Read the model definition and answer for the solid it produces. Units are mm, in the model's axes. Give positions to 0.01 mm unless a question says otherwise; leave off trailing zeros. Order: outer loops, then holes, each group sorted by start corner. A loop starts at its lowest first (then second) coordinate and runs counter-clockwise, first axis right, second up. Notation, with made-up numbers: (-22.75, 74) - (-8.75, 74) arc R18 cw to (-8.75, 89) - close; hole circle Ø4 at (76.5, 62). An arc over 180 degrees is marked (long way). Write each question's results on one line, items separated by ' | '. Start each with the question number.
Q1. Find section C-C on x = 25.5. Give the vertices of the cut face in (y, z).
Q2. Find the intervals of material crossed by line 1 along Z through (x, y) = (-41.5, 1.1); line 2 along X through (y, z) = (0.3, -42); line 3 along X through (y, z) = (1.55, -26), in increasing order. Write a range as from..to.
Q3. Flat-ended cylindrical pins translate along their axes: P1, Ø1, axis at y = 4, z = -29, coming from the -X side; P2, Ø1.5, axis at y = 2, z = -28.5, coming from the +X side; P3, Ø3, axis at x = -17, y = 3.5, coming from the +Z side. Find the tip coordinate at first contact, or state that the pin passes through.
Q4. Find section B-B on z = 38.5. Give the vertices of the cut face in (x, y), and give its area (3 significant figures).
Q5. Find section A-A on y = 3.7. Count the separate pieces of the cut face and the enclosed holes in it, and give its area (3 significant figures).
from build123d import *

# Parameters (mm, degrees)
BOSS_EXTRUDE2_DEPTH = 5
FILLET2_R           = 5
SKETCH4_R           = 2.25
CUT_EXTRUDE1_DEPTH  = 68.360967927


with BuildPart() as part:
    # Sketch3 → Boss-Extrude2 (new body)
    with BuildSketch(Plane(origin=(0, 0, 0), x_dir=(1, 0, 0), z_dir=(0, 1, 0))):
        with BuildLine():
            Line((-32.880465325, -20.152543264), (-39.343121117, -26.615199056))
            ThreePointArc((-39.343121117, -26.615199056), (-37.337514667, -29.36256117), (-35.140434727, -31.95934679))
            ThreePointArc((-35.140434727, -31.95934679), (-32.701976515, -31.519186154), (-31.337572106, -33.587572106))
            ThreePointArc((-31.337572106, -33.587572106), (-31.498791725, -34.423931191), (-31.95934679, -35.140434727))
            ThreePointArc((-31.95934679, -35.140434727), (-29.36256117, -37.337514667), (-26.615199056, -39.343121117))
            Line((-26.615199056, -39.343121117), (-20.152543264, -32.880465325))
            Line((-20.152543264, -32.880465325), (-32.880465325, -20.152543264))
        make_face()
        with BuildLine():
            ThreePointArc((-35.140434727, -31.95934679), (-37.337514667, -29.36256117), (-39.343121117, -26.615199056))
            Line((-39.343121117, -26.615199056), (-42.072853481, -29.344931419))
            ThreePointArc((-42.072853481, -29.344931419), (-43.537319575, -32.880465325), (-42.072853481, -36.415999231))
            Line((-42.072853481, -36.415999231), (-36.415999231, -42.072853481))
            ThreePointArc((-36.415999231, -42.072853481), (-32.880465325, -43.537319575), (-29.344931419, -42.072853481))
            Line((-29.344931419, -42.072853481), (-26.615199056, -39.343121117))
            ThreePointArc((-26.615199056, -39.343121117), (-29.36256117, -37.337514667), (-31.95934679, -35.140434727))
            ThreePointArc((-31.95934679, -35.140434727), (-35.178562364, -35.178562364), (-35.140434727, -31.95934679))
        make_face()
        with BuildLine():
            Line((42.072853481, -29.344931419), (39.343121117, -26.615199056))
            ThreePointArc((39.343121117, -26.615199056), (37.337514667, -29.36256117), (35.140434727, -31.95934679))
            ThreePointArc((35.140434727, -31.95934679), (35.655958059, -32.701976515), (35.837572106, -33.587572106))
            ThreePointArc((35.837572106, -33.587572106), (34.423931191, -35.676352488), (31.95934679, -35.140434727))
            ThreePointArc((31.95934679, -35.140434727), (29.36256117, -37.337514667), (26.615199056, -39.343121117))
            Line((26.615199056, -39.343121117), (29.344931419, -42.072853481))
            ThreePointArc((29.344931419, -42.072853481), (32.880465325, -43.537319575), (36.415999231, -42.072853481))
            Line((36.415999231, -42.072853481), (42.072853481, -36.415999231))
            ThreePointArc((42.072853481, -36.415999231), (43.537319575, -32.880465325), (42.072853481, -29.344931419))
        make_face()
        with BuildLine():
            Line((-20.152543264, 32.880465325), (-26.615199056, 39.343121117))
            ThreePointArc((-26.615199056, 39.343121117), (-29.36256117, 37.337514667), (-31.95934679, 35.140434727))
            ThreePointArc((-31.95934679, 35.140434727), (-31.498791725, 34.423931191), (-31.337572106, 33.587572106))
            ThreePointArc((-31.337572106, 33.587572106), (-32.701976515, 31.519186154), (-35.140434727, 31.95934679))
            ThreePointArc((-35.140434727, 31.95934679), (-37.337514667, 29.36256117), (-39.343121117, 26.615199056))
            Line((-39.343121117, 26.615199056), (-32.880465325, 20.152543264))
            Line((-32.880465325, 20.152543264), (-20.152543264, 32.880465325))
        make_face()
        with BuildLine():
            ThreePointArc((-31.95934679, 35.140434727), (-29.36256117, 37.337514667), (-26.615199056, 39.343121117))
            Line((-26.615199056, 39.343121117), (-29.344931419, 42.072853481))
            ThreePointArc((-29.344931419, 42.072853481), (-32.880465325, 43.537319575), (-36.415999231, 42.072853481))
            Line((-36.415999231, 42.072853481), (-42.072853481, 36.415999231))
            ThreePointArc((-42.072853481, 36.415999231), (-43.537319575, 32.880465325), (-42.072853481, 29.344931419))
            Line((-42.072853481, 29.344931419), (-39.343121117, 26.615199056))
            ThreePointArc((-39.343121117, 26.615199056), (-37.337514667, 29.36256117), (-35.140434727, 31.95934679))
            ThreePointArc((-35.140434727, 31.95934679), (-35.178562364, 35.178562364), (-31.95934679, 35.140434727))
        make_face()
        with BuildLine():
            Line((20.152543264, 32.880465325), (26.615199056, 39.343121117))
            ThreePointArc((26.615199056, 39.343121117), (0, 47.5), (-26.615199056, 39.343121117))
            Line((-26.615199056, 39.343121117), (-20.152543264, 32.880465325))
            Line((-20.152543264, 32.880465325), (-32.880465325, 20.152543264))
            Line((-32.880465325, 20.152543264), (-39.343121117, 26.615199056))
            ThreePointArc((-39.343121117, 26.615199056), (-47.5, 0), (-39.343121117, -26.615199056))
            Line((-39.343121117, -26.615199056), (-32.880465325, -20.152543264))
            Line((-32.880465325, -20.152543264), (-20.152543264, -32.880465325))
            Line((-20.152543264, -32.880465325), (-26.615199056, -39.343121117))
            ThreePointArc((-26.615199056, -39.343121117), (0, -47.5), (26.615199056, -39.343121117))
            Line((26.615199056, -39.343121117), (20.152543264, -32.880465325))
            Line((20.152543264, -32.880465325), (32.880465325, -20.152543264))
            Line((32.880465325, -20.152543264), (39.343121117, -26.615199056))
            ThreePointArc((39.343121117, -26.615199056), (45.415020935, -13.91854423), (47.5, 0))
            ThreePointArc((47.5, 0), (45.415020935, 13.91854423), (39.343121117, 26.615199056))
            Line((39.343121117, 26.615199056), (32.880465325, 20.152543264))
            Line((32.880465325, 20.152543264), (20.152543264, 32.880465325))
        make_face()
        with BuildLine():
            Line((42.072853481, 36.415999231), (36.415999231, 42.072853481))
            ThreePointArc((36.415999231, 42.072853481), (32.880465325, 43.537319575), (29.344931419, 42.072853481))
            Line((29.344931419, 42.072853481), (26.615199056, 39.343121117))
            ThreePointArc((26.615199056, 39.343121117), (29.36256117, 37.337514667), (31.95934679, 35.140434727))
            ThreePointArc((31.95934679, 35.140434727), (34.423931191, 35.676352488), (35.837572106, 33.587572106))
            ThreePointArc((35.837572106, 33.587572106), (35.655958059, 32.701976515), (35.140434727, 31.95934679))
            ThreePointArc((35.140434727, 31.95934679), (37.337514667, 29.36256117), (39.343121117, 26.615199056))
            Line((39.343121117, 26.615199056), (42.072853481, 29.344931419))
            ThreePointArc((42.072853481, 29.344931419), (43.537319575, 32.880465325), (42.072853481, 36.415999231))
        make_face()
        with BuildLine():
            ThreePointArc((31.95934679, 35.140434727), (29.36256117, 37.337514667), (26.615199056, 39.343121117))
            Line((26.615199056, 39.343121117), (20.152543264, 32.880465325))
            Line((20.152543264, 32.880465325), (32.880465325, 20.152543264))
            Line((32.880465325, 20.152543264), (39.343121117, 26.615199056))
            ThreePointArc((39.343121117, 26.615199056), (37.337514667, 29.36256117), (35.140434727, 31.95934679))
            ThreePointArc((35.140434727, 31.95934679), (31.996581849, 31.996581849), (31.95934679, 35.140434727))
        make_face()
        with BuildLine():
            ThreePointArc((35.140434727, -31.95934679), (37.337514667, -29.36256117), (39.343121117, -26.615199056))
            Line((39.343121117, -26.615199056), (32.880465325, -20.152543264))
            Line((32.880465325, -20.152543264), (20.152543264, -32.880465325))
            Line((20.152543264, -32.880465325), (26.615199056, -39.343121117))
            ThreePointArc((26.615199056, -39.343121117), (29.36256117, -37.337514667), (31.95934679, -35.140434727))
            ThreePointArc((31.95934679, -35.140434727), (31.996581849, -31.996581849), (35.140434727, -31.95934679))
        make_face()
    extrude(amount=BOSS_EXTRUDE2_DEPTH)

    # Fillet2
    # the kernel refuses this fillet: 5 mm, written as the material it adds along each edge
    with BuildSketch(Plane(origin=(39.343121117, 0, -26.615199056), x_dir=(0.7070624227477131, 0, -0.7071511368428492), z_dir=(0, 1, 0)), Plane(origin=(26.615199056, 0, 39.343121117), x_dir=(0.7071511368428588, 0, 0.7070624227477036), z_dir=(0, 1, 0)), Plane(origin=(-39.343121117, 0, 26.615199056), x_dir=(-0.7070624227477083, 0, 0.7071511368428542), z_dir=(0, 1, 0))) as fillet2_piece_1:
        with BuildLine():
            CenterArc((3.959159658, -4.999757824), FILLET2_R, 90.563922665, 73.967028667)
            Line((-0.85971372, -3.666168917), (-1.341601058, -3.532810027))
            ThreePointArc((-1.341601058, -3.532810027), (-0.880307289, -1.727454188), (-0.490936956, 0.094767639))
            Line((-0.490936956, 0.094767639), (3.1365e-05, 0.499999999))
            ThreePointArc((3.1365e-05, 0.499999999), (3.860455888, 0.499757833), (3.905027842, 0.499975782))
            Line((3.905027842, 0.499975782), (3.909948916, 0))
        make_face()
    extrude(amount=5)
    with BuildSketch(Plane(origin=(39.343121117, 0, 26.615199056), x_dir=(0.5270483151483139, 0, -0.849835321400166), z_dir=(0, 1, 0)), Plane(origin=(-26.615199056, 0, 39.343121117), x_dir=(0.8498353214001645, 0, 0.5270483151483165), z_dir=(0, 1, 0)), Plane(origin=(26.615199056, 0, -39.343121117), x_dir=(-0.8498353214001678, 0, -0.5270483151483113), z_dir=(0, 1, 0))) as fillet2_piece_2:
        with BuildLine():
            CenterArc((3.963811676, -4.996070505), FILLET2_R, 92.271691936, 73.967028667)
            Line((-0.892664621, -3.806684962), (-1.378312251, -3.687746408))
            ThreePointArc((-1.378312251, -3.687746408), (-1.367924016, -3.644401383), (-0.486801878, 0.11412244))
            Line((-0.486801878, 0.11412244), (0.019819058, 0.499607051))
            ThreePointArc((0.019819058, 0.499607051), (1.882810546, 0.462669799), (3.745802034, 0.499607051))
            Line((3.745802034, 0.499607051), (3.765621092, 0))
        make_face()
    extrude(amount=5)
    with BuildSketch(Plane(origin=(-39.343121117, 0, -26.615199056), x_dir=(-0.7070624227477041, 0, -0.7071511368428584), z_dir=(0, 1, 0))) as fillet2_piece_3:
        with BuildLine():
            CenterArc((3.959159658, 4.999757824), FILLET2_R, 195.469048668, 73.967028667)
            Line((-0.85971372, 3.666168917), (-1.341601058, 3.532810027))
            ThreePointArc((-1.341601058, 3.532810027), (-0.880307289, 1.727454188), (-0.490936956, -0.094767639))
            Line((-0.490936956, -0.094767639), (3.1365e-05, -0.499999999))
            ThreePointArc((3.1365e-05, -0.499999999), (3.860455888, -0.499757833), (3.905027842, -0.499975782))
            Line((3.905027842, -0.499975782), (3.909948916, 0))
        make_face()
    extrude(amount=5)
    with BuildSketch(Plane(origin=(-26.615199056, 0, -39.343121117), x_dir=(0.8498353214001803, 0, -0.527048315148291), z_dir=(0, 1, 0))) as fillet2_piece_4:
        with BuildLine():
            CenterArc((3.963811676, 4.996070505), FILLET2_R, 193.761279397, 73.967028667)
            Line((-0.892664621, 3.806684962), (-1.378312251, 3.687746408))
            ThreePointArc((-1.378312251, 3.687746408), (-1.367924016, 3.644401383), (-0.486801878, -0.11412244))
            Line((-0.486801878, -0.11412244), (0.019819058, -0.499607051))
            ThreePointArc((0.019819058, -0.499607051), (1.882810546, -0.462669799), (3.745802034, -0.499607051))
            Line((3.745802034, -0.499607051), (3.765621092, 0))
        make_face()
    extrude(amount=5)
    # the kernel refuses this fillet: 5 mm, written as the material it takes off along each edge

    # Sketch4 → Cut-Extrude1 (cut, through all)
    with BuildSketch(Plane(origin=(0, 5, 0), x_dir=(1, 0, 0), z_dir=(0, 1, 0))):
        with Locations(Location((-20.882726769, -12.213969589, 0), (0, 0, 270))):
            Circle(SKETCH4_R)
        with Locations(Location((-4.308326491, 26.840982151, 0), (0, 0, 270))):
            Circle(SKETCH4_R)
        with Locations(Location((34.746625249, 10.266581873, 0), (0, 0, 270))):
            Circle(SKETCH4_R)
        with Locations(Location((18.172224972, -28.788369867, 0), (0, 0, 270))):
            Circle(SKETCH4_R)
    extrude(amount=-CUT_EXTRUDE1_DEPTH, mode=Mode.SUBTRACT)


solid = part.part
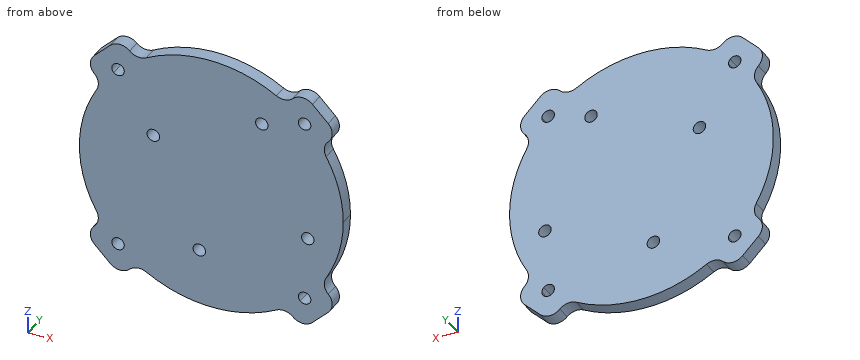
Working result:
1) outline: (0, -40.69) - (5, -40.69) - (5, 40.69) - (0, 40.69) - close
2) line 1: -36.99..-28.63, -23.11..23.11, 28.63..36.99 | line 2: -36.49..-29.27, -22.19..22.19, 29.27..36.49 | line 3: -40.68..-6.4, -2.22..40.68
3) P1: x = -42.22 | P2: x = 41.98 | P3: z = 44.9
4) outline: (-39.99, 0) - (39.99, 0) - (39.99, 5) - (-39.99, 5) - close | area: 400 mm²
5) separate pieces: 1 | enclosed holes: 8 | area: 7,540 mm²
